Can you work these out from the model? Positions are in its coordinate system, mm. A direction names the side the tool comes from. Coordinates: 2 decimals unless noted, no trailing zeros. Order: outer loops, then holes, each group sorted by start corner. A loop starts at its lowest first (then second) coordinate and runs counter-clockwise, first axis right, second up. Notation, with made-up numbers: (-28, -29) -> (0, -29) arc R35 ccw to (0, 8) -> close; hole circle Ø7 at (-11.75, 54). An arc over 180 degrees is marked (long way). Use a Markdown table: item, result. Add a question column.
1. For pin 1 Ø3.5 at (x, z) = (-5, 35) entering from -Y; pin 2 Ø4 at (x, z) = (-59, 35) entering from +Y; pin 3 Ø0.6 at (x, z) = (-62.5, 18.5) entering from -Y, each with a flat end and sliding along its axis, tell me the tip position at first contact or that it passes through.
2. Suppose I cut it at B-B, the plane y = 36. List the corners of the cut face in (x, z) for me, then the cut area to 3 significant figures.
3. For faces 1 (the flat face through (-1, 28.629, 20)), 2 (the flat face through (-64, 42, 20)), 3 (the flat face through (-62, 36, 20)), which set-ups out of +Z, -Z, +X, -X, +Y, -Y let a thin tool reach every point of the face, with its end or its side?
4. Suppose I cut it at D-D, the plane x = -21. List the corners of the cut face in (y, z) for me.
5. Suppose I cut it at A-A, the plane x = -5. List the corners of the cut face in (y, z) for me, then the cut area to 3 significant figures.
6. If I drill on line 1 along X through (y, z) = (1, 35); line 2 along X through (y, z) = (32, 26); line 3 along Y through (x, z) = (-57, 35), over which ranges is the centre line in solid material (lowest first)? Write a range as from..to.
7. Suppose I cut it at C-C, the plane y = 12. List the corners of the cut face in (x, z) for me.
8. We'd pull the mould along Z, two halves only. Please class faces 4 (the flat face through (-32, 2, 35)), 5 (the flat face through (-32, 1, 40)), 6 (the cylindrical face through (-1.01, 66.99, 2.85)), 7 (the cylindrical face through (-5.9, 1, 36.2)): pulls with the +Z half, pulls with the -Z half, needs draft (parallel to the pull), parting line crosses it, or undercut.
```python
from build123d import *

# Parameters (mm, degrees)
EXTRUDE_THIN1_DEPTH = 40
CUT_EXTRUDE2_DEPTH  = 60
FILLET1_R           = 10
SKETCH3_R           = 1.5
CUT_EXTRUDE4_DEPTH  = 20


with BuildPart() as part:
    # Sketch1 → Extrude-Thin1 (new body)
    with BuildSketch(Plane.XY):
        Polygon((-32, 0), (0, 0), (0, 70), (-2, 70), (-2, 2), (-32, 2), align=None)
    extrude(amount=EXTRUDE_THIN1_DEPTH)

    # Sketch2 → Cut-Extrude2 (cut)
    with BuildSketch(Plane(origin=(0, 0, 0), x_dir=(0, 0, -1), z_dir=(1, 0, 0))):
        with BuildLine():
            ThreePointArc((-20, 62.5), (-27.5, 55), (-20, 47.5))
            Line((-20, 47.5), (-20, 62.5))
        make_face()
        with BuildLine():
            Line((-20, 62.5), (-20, 47.5))
            ThreePointArc((-20, 47.5), (-14.696699141, 49.696699141), (-12.5, 55))
            ThreePointArc((-12.5, 55), (-14.696699141, 60.303300859), (-20, 62.5))
        make_face()
        with BuildLine():
            Line((-9.327670915, 25), (-9.327670915, 0))
            Line((-9.327670915, 0), (-31.039452712, 0))
            Line((-31.039452712, 0), (-31.039452712, 25))
            ThreePointArc((-31.039452712, 25), (-29.976608153, 27.56593375), (-27.410674402, 28.62877831))
            Line((-27.410674402, 28.62877831), (-12.956449225, 28.62877831))
            ThreePointArc((-12.956449225, 28.62877831), (-10.390515474, 27.56593375), (-9.327670915, 25))
        make_face()
    extrude(amount=-CUT_EXTRUDE2_DEPTH, mode=Mode.SUBTRACT)

    # Fillet1
    fillet1_edges = [part.edges().sort_by_distance(p)[0] for p in [
        (-1, 70, 0),
        (-1, 70, 40),
    ]]
    fillet(fillet1_edges, radius=FILLET1_R)

    # Mirror1: part across plane


with BuildPart() as part_1:
    add(part.part)
    add(part.part.mirror(Plane(origin=(-32, 0, 40), x_dir=(0, 0, 1), z_dir=(-1, 0, 0))))

    # Sketch3 → Cut-Extrude4 (cut)
    with BuildSketch(Plane.XZ):
        with Locations(Location((-59, 35, 0), (0, 0, 270))):
            Circle(SKETCH3_R)
        with Locations(Location((-5, 35, 0), (0, 0, 270))):
            Circle(SKETCH3_R)
        with Locations(Location((-5, 5, 0), (0, 0, 270))):
            Circle(SKETCH3_R)
        with Locations(Location((-59, 5, 0), (0, 0, 270))):
            Circle(SKETCH3_R)
    extrude(amount=-CUT_EXTRUDE4_DEPTH, mode=Mode.SUBTRACT)


solid = part_1.part
```
Worked out:
| question | item | result |
|---|---|---|
| 1 | pin 1 | stops at y = 0 |
| 1 | pin 2 | stops at y = 2 |
| 1 | pin 3 | stops at y = 28.63 |
| 2 | outline | (-64, 0) -> (-62, 0) -> (-62, 40) -> (-64, 40) -> close; (-2, 0) -> (0, 0) -> (0, 40) -> (-2, 40) -> close |
| 2 | area | 160 mm² |
| 3 | face 1 | +X, -X, -Y |
| 3 | face 2 | +Z, -Z, -X, +Y, -Y |
| 3 | face 3 | +Z, -Z, +Y |
| 4 | outline | (0, 0) -> (2, 0) -> (2, 9.33) -> (0, 9.33) -> close; (0, 31.04) -> (2, 31.04) -> (2, 40) -> (0, 40) -> close |
| 5 | outline | (0, 0) -> (2, 0) -> (2, 3.5) -> (0, 3.5) -> close; (0, 6.5) -> (2, 6.5) -> (2, 9.33) -> (0, 9.33) -> close; (0, 31.04) -> (2, 31.04) -> (2, 33.5) -> (0, 33.5) -> close; (0, 36.5) -> (2, 36.5) -> (2, 40) -> (0, 40) -> close |
| 5 | area | 24.6 mm² |
| 6 | line 1 | x = -64..-60.5, -57.5..-6.5, -3.5..0 |
| 6 | line 2 | x = -64..-62, -2..0 |
| 6 | line 3 | y = 0..2 |
| 7 | outline | (-64, 0) -> (-62, 0) -> (-62, 9.33) -> (-64, 9.33) -> close; (-64, 31.04) -> (-62, 31.04) -> (-62, 40) -> (-64, 40) -> close; (-2, 0) -> (0, 0) -> (0, 9.33) -> (-2, 9.33) -> close; (-2, 31.04) -> (0, 31.04) -> (0, 40) -> (-2, 40) -> close |
| 8 | face 4 | needs draft |
| 8 | face 5 | pulls with the +Z half |
| 8 | face 6 | pulls with the -Z half |
| 8 | face 7 | undercut |
